Check sheet for the drawn part. Datum: minimum x, y, z corner. Units: mm. A direction names the side the tool comes from. Coordinates: 2 decimals unless noted, no trailing zeros. Loops run counter-clockwise (first coordinate to the right, second up) from the corner with the lowest first, then second, coordinate; pieces in that order, holes last. Notation, with made-up numbers: (43, 7.25) - (89, 7.25) arc R19 cw to (89, 44.25) - close; hole circle Ø7 at (81.5, 14.5). An arc over 180 degrees is marked (long way). Answer as CSV lines item,"result". Start each with the question number.
1. Set-up check for the marked faces 1 and 2: record each of +Z, -Z, +X, -X, +Y, -Y from which the full face is reachable in a straight line by a thin tool's end or side.
2. Material ranges on line 1 (Y direction, x = 0.6, z = 1.8); line 2 (Z direction, x = 2.55, y = 17); line 3 (Z direction, x = 4.1, y = 20) (1 decimal), recorded low to high. Write a range as [from, to].
3. Cross-section at A-A (y = 14.75). Enter the section's corners in (x, z).
4. Gauge pin test, flat ends, axial feed: P1, Ø1.5, axis at x = 4.5, y = 9, coming from the -Z side (1 decimal); P2, Ø1, axis at x = 2, y = 8.5, coming from the -Z side; P3, Ø2, axis at y = 19, z = 2.5, coming from the -X side. Record the tip position at first contact, or that the pin passes through.
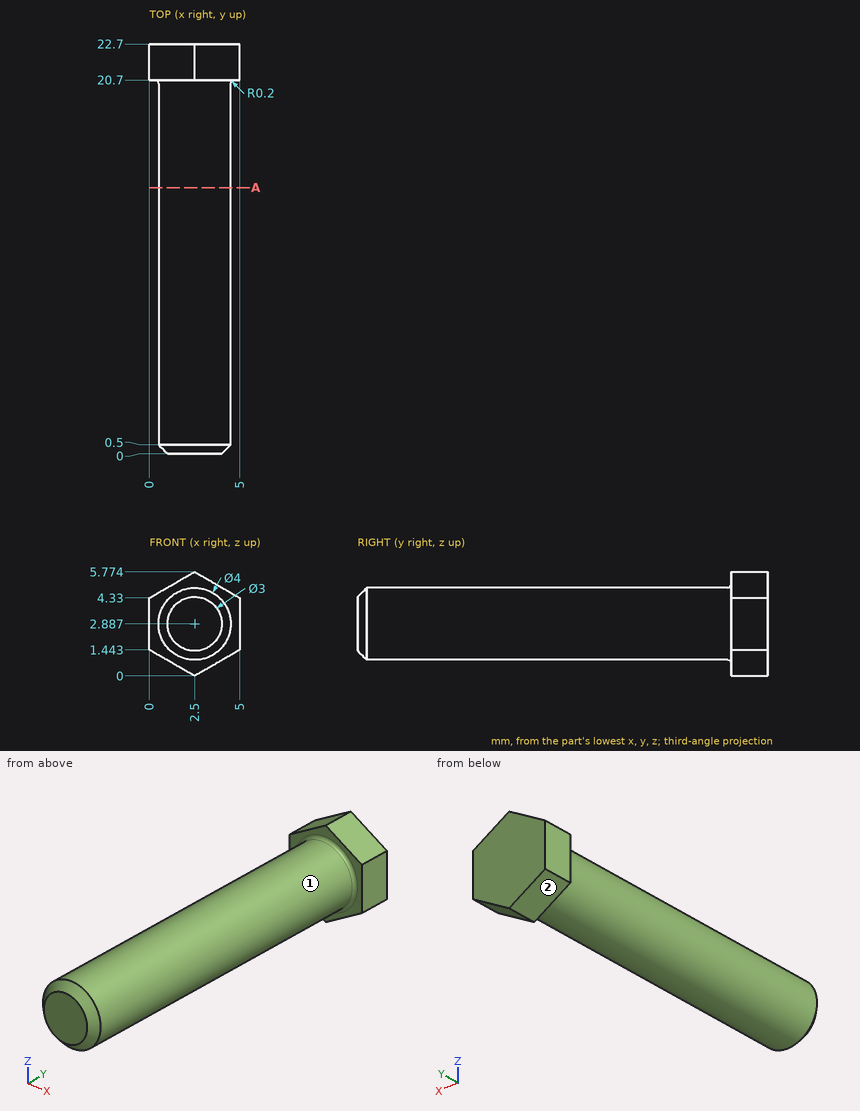
Values follow:
1,face 1,"-Y"
1,face 2,"-Z, -X, +Y, -Y"
2,line 1,"y = [20.7, 22.7]"
2,line 2,"z = [0.89, 4.89]"
2,line 3,"z = [1.7, 4.1]"
3,outline,"circle Ø4 at (2.5, 2.89)"
4,P1,"stops at z = 1.3"
4,P2,"stops at z = 0.89"
4,P3,"stops at x = 0.5"
